from build123d import *

# Parameters (mm, degrees)
CROQUIS1_W              = 35
CROQUIS1_H              = 120
SALIENTE_EXTRUIR1_DEPTH = 6
CROQUIS3_W              = 6.02
CROQUIS3_H              = 40.02
CORTAR_EXTRUIR1_DEPTH   = 126.143917151
CROQUIS4_W              = 6.05
CROQUIS4_H              = 80
CORTAR_EXTRUIR2_DEPTH   = 10
CROQUIS5_W              = 21
CROQUIS5_H              = 7
SALIENTE_EXTRUIR2_DEPTH = 6


with BuildPart() as part:
    # Croquis1 → Saliente-Extruir1 (new body)
    with BuildSketch(Plane(origin=(0, 0, 0), x_dir=(0, 0, -1), z_dir=(1, 0, 0))):
        with Locations((17.5, 60)):
            Rectangle(CROQUIS1_W, CROQUIS1_H)
    extrude(amount=SALIENTE_EXTRUIR1_DEPTH)

    # Croquis3 → Cortar-Extruir1 (cut, through all)
    with BuildSketch(Plane(origin=(0, 0, 0), x_dir=(0, 0, -1), z_dir=(1, 0, 0))):
        with Locations((31.99, 60)):
            Rectangle(CROQUIS3_W, CROQUIS3_H)
    extrude(amount=CORTAR_EXTRUIR1_DEPTH, mode=Mode.SUBTRACT)

    # Croquis4 → Cortar-Extruir2 (cut)
    with BuildSketch(Plane(origin=(0, 0, 0), x_dir=(0, 0, -1), z_dir=(1, 0, 0))):
        with Locations((10.955, 60)):
            Rectangle(CROQUIS4_W, CROQUIS4_H)
    extrude(amount=CORTAR_EXTRUIR2_DEPTH, mode=Mode.SUBTRACT)

    # Croquis5 → Saliente-Extruir2 (add)
    with BuildSketch(Plane(origin=(0, 0, 0), x_dir=(0, 0, -1), z_dir=(1, 0, 0))):
        with Locations((10.5, 123.5)):
            Rectangle(CROQUIS5_W, CROQUIS5_H)
    extrude(amount=SALIENTE_EXTRUIR2_DEPTH)


solid = part.part
Design review of the part built by this model. Coordinates are the model's own, in mm. A direction names the side the tool comes from. Round coordinates to 2 decimals unless told otherwise and drop trailing zeros. Write each loop counter-clockwise with the first axis right and the second up, starting at its lowest first coordinate (ties: lowest second). Pieces come first, ordered by that corner, then holes.
Item 1: Consider section A-A on x = 1.6. Give the boundary of the cut face in (y, z), and give its area (3 significant figures).
Item 2: Wall thickness on L1, parallel to Z at x = 4.2, y = 82.5; L2, parallel to Z at x = 1.75, y = 75.5; L3, parallel to Y at x = 3.9, z = -11.5: over which ranges is each line inside the solid? List them lowest first.
Item 3: Draft analysis for pull direction Y (two halves, no side actions). For faces 1 (the flat face through (3, 20, -35)), 2 (the flat face through (3, 120, -28)), 3 (the flat face through (3, 80.01, -32)), state which applies: released by +Y, released by -Y, zero draft, split by the parting line, or undercut.
Item 4: Consider section C-C on y = 34. Give the boundary of the cut face in (x, z).
Item 5: For faces 4 (the flat face through (3, 39.99, -32)), 5 (the flat face through (3, 127, -10)), 6 (the flat face through (3, 59, -7.93)), 7 (the flat face through (3, 123, -21)), 8 (the flat face through (3, 63, 0)), list the 3-axis set-ups (+Z, -Z, +X, -X, +Y, -Y) from which the entire face can be reached by the end or side of a thin tool; tool diameter is ignored.
Item 6: Consider section B-B on z = -32. Give the boundary of the cut face in (x, y).
Item 7: Consider section D-D on z = -26. Give the boundary of the cut face in (x, y), and give its area (3 significant figures).
Item 8: For pin 1 Ø3 at (x, z) = (2, -32) entering from +Y; pin 2 Ø1.8 at (x, y) = (3, 123.5) entering from -Z; pin 3 Ø3 at (x, y) = (4.5, 53.5) entering from -Z, all flat-tipped, find the tip position at first contact; note any pin that passes through.
Check values:
1. outline: (0, -35) - (39.99, -35) - (39.99, -28.98) - (80.01, -28.98) - (80.01, -35) - (120, -35) - (120, -21) - (127, -21) - (127, 0) - (0, 0) - close; hole (20, -13.98) - (100, -13.98) - (100, -7.93) - (20, -7.93) - close
1. area: 3,620 mm2
2. L1: z = -35 to -13.98, -7.93 to 0
2. L2: z = -28.98 to -13.98, -7.93 to 0
2. L3: y = 0 to 20, 100 to 127
3. face 1: zero draft
3. face 2: released by +Y
3. face 3: undercut
4. outline: (0, -35) - (6, -35) - (6, -13.98) - (0, -13.98) - close; (0, -7.93) - (6, -7.93) - (6, 0) - (0, 0) - close
5. face 4: -Z, +X, -X
5. face 5: +Z, -Z, +X, -X, +Y
5. face 6: +X, -X
5. face 7: -Z, +X, -X, +Y
5. face 8: +Z, +X, -X, +Y, -Y
6. outline: (0, 0) - (6, 0) - (6, 39.99) - (0, 39.99) - close; (0, 80.01) - (6, 80.01) - (6, 120) - (0, 120) - close
7. outline: (0, 0) - (6, 0) - (6, 120) - (0, 120) - close
7. area: 720 mm2
8. pin 1: stops at y = 120
8. pin 2: stops at z = -21
8. pin 3: stops at z = -28.98
